```python
from build123d import *

# Parameters (mm, degrees)
F1_DEPTH = 21.6916
F3_DEPTH = 2
F0_R     = 3.175
F4_DEPTH = 2


with BuildPart() as f1:
    # F0 (on Top) → F1 (new body)
    with BuildSketch(Plane.XY):
        Polygon((-7.366008, 32.2749), (-13.577315, 21.5166), (-7.366008, 10.7583), (-13.577315, 0), (-6.788658, -11.7583), (6.788658, -11.7583), (12.999965, -1), (24.267879, -1), (30.479187, -11.7583), (44.056502, -11.7583), (50.267809, -1), (62.690424, -1), (69.479082, 10.7583), (63.267775, 21.5166), (69.479082, 32.2749), (63.267775, 43.0332), (69.479082, 53.7915), (62.690424, 65.5498), (49.113109, 65.5498), (42.901802, 54.7915), (31.633887, 54.7915), (25.42258, 65.5498), (11.845265, 65.5498), (5.633957, 54.7915), (-6.788658, 54.7915), (-13.577315, 43.0332), align=None)
        Polygon((-5.633957, 9.7583), (5.633957, 9.7583), (11.267914, 0), (5.633957, -9.7583), (-5.633957, -9.7583), (-11.267914, 0), align=None, mode=Mode.SUBTRACT)
        Polygon((11.267914, 21.5166), (5.633957, 11.7583), (-5.633957, 11.7583), (-11.267914, 21.5166), (-5.633957, 31.2749), (5.633957, 31.2749), align=None, mode=Mode.SUBTRACT)
        Polygon((12.999965, 20.5166), (24.267879, 20.5166), (29.901836, 10.7583), (24.267879, 1), (12.999965, 1), (7.366008, 10.7583), align=None, mode=Mode.SUBTRACT)
        Polygon((48.535759, 0), (42.901802, -9.7583), (31.633887, -9.7583), (25.99993, 0), (31.633887, 9.7583), (42.901802, 9.7583), align=None, mode=Mode.SUBTRACT)
        Polygon((25.99993, 21.5166), (31.633887, 31.2749), (42.901802, 31.2749), (48.535759, 21.5166), (42.901802, 11.7583), (31.633887, 11.7583), align=None, mode=Mode.SUBTRACT)
        Polygon((61.535724, 1), (50.267809, 1), (44.633852, 10.7583), (50.267809, 20.5166), (61.535724, 20.5166), (67.169681, 10.7583), align=None, mode=Mode.SUBTRACT)
        Polygon((11.267914, 43.0332), (5.633957, 33.2749), (-5.633957, 33.2749), (-11.267914, 43.0332), (-5.633957, 52.7915), (5.633957, 52.7915), align=None, mode=Mode.SUBTRACT)
        Polygon((24.267879, 22.5166), (12.999965, 22.5166), (7.366008, 32.2749), (12.999965, 42.0332), (24.267879, 42.0332), (29.901836, 32.2749), align=None, mode=Mode.SUBTRACT)
        Polygon((24.267879, 44.0332), (12.999965, 44.0332), (7.366008, 53.7915), (12.999965, 63.5498), (24.267879, 63.5498), (29.901836, 53.7915), align=None, mode=Mode.SUBTRACT)
        Polygon((25.99993, 43.0332), (31.633887, 52.7915), (42.901802, 52.7915), (48.535759, 43.0332), (42.901802, 33.2749), (31.633887, 33.2749), align=None, mode=Mode.SUBTRACT)
        Polygon((67.169681, 32.2749), (61.535724, 22.5166), (50.267809, 22.5166), (44.633852, 32.2749), (50.267809, 42.0332), (61.535724, 42.0332), align=None, mode=Mode.SUBTRACT)
        Polygon((50.267809, 63.5498), (61.535724, 63.5498), (67.169681, 53.7915), (61.535724, 44.0332), (50.267809, 44.0332), (44.633852, 53.7915), align=None, mode=Mode.SUBTRACT)
    extrude(amount=F1_DEPTH)

    # F2 (on face) → F3 (join)
    with BuildSketch(Plane(origin=(0, 0, 0), x_dir=(1, 0, 0), z_dir=(0, 0, -1))):
        Polygon((69.479082, -53.7915), (63.267775, -43.0332), (69.479082, -32.2749), (63.267775, -21.5166), (69.479082, -10.7583), (62.690424, 1), (50.267809, 1), (44.056502, 11.7583), (30.479187, 11.7583), (24.267879, 1), (12.999965, 1), (6.788658, 11.7583), (-6.788658, 11.7583), (-13.577315, 0), (-7.366008, -10.7583), (-13.577315, -21.5166), (-7.366008, -32.2749), (-13.577315, -43.0332), (-6.788658, -54.7915), (5.633957, -54.7915), (11.845265, -65.5498), (25.42258, -65.5498), (31.633887, -54.7915), (42.901802, -54.7915), (49.113109, -65.5498), (62.690424, -65.5498), align=None)
    extrude(amount=F3_DEPTH)

    # F0 (on Top) → F4 (cut, through all)
    with BuildSketch(Plane.XY):
        with Locations((0, 43.0332)):
            Circle(F0_R)
        with Locations((18.633922, 53.7915)):
            Circle(F0_R)
        with Locations((37.267844, 43.0332)):
            Circle(F0_R)
        with Locations((55.901767, 53.7915)):
            Circle(F0_R)
        with Locations((55.901767, 32.2749)):
            Circle(F0_R)
        with Locations((37.267844, 21.5166)):
            Circle(F0_R)
        with Locations((18.633922, 32.2749)):
            Circle(F0_R)
        with Locations((0, 21.5166)):
            Circle(F0_R)
        Circle(F0_R)
        with Locations((18.633922, 10.7583)):
            Circle(F0_R)
        with Locations((37.267844, 0)):
            Circle(F0_R)
        with Locations((55.901767, 10.7583)):
            Circle(F0_R)
    extrude(amount=-F4_DEPTH, mode=Mode.SUBTRACT)


solid = f1.part
```
Verification items for the finished model (mm, model axes). A direction names the side the tool comes from. Round coordinates to 2 decimals unless told otherwise and drop trailing zeros. Loops run counter-clockwise (first coordinate to the right, second up) from the corner with the lowest first, then second, coordinate; pieces in that order, holes last. Notation, with made-up numbers: (2.25, 50.25) -> (9.25, 50.25) arc R21 ccw to (9.25, 81.25) -> close; hole circle Ø7 at (-23.75, 38.5). An arc over 180 degrees is marked (long way). Answer as a JSON object with one key per item and string values.
Q1. Section check A-A (x = 0). Record the boundary of the cut face in (y, z) (1 decimal).
Data:
{"outline": "(-11.8, -2) -> (-3.2, -2) -> (-3.2, 0) -> (-9.8, 0) -> (-9.8, 21.7) -> (-11.8, 21.7) -> close; (3.2, -2) -> (18.3, -2) -> (18.3, 0) -> (11.8, 0) -> (11.8, 21.7) -> (9.8, 21.7) -> (9.8, 0) -> (3.2, 0) -> close; (24.7, -2) -> (39.9, -2) -> (39.9, 0) -> (33.3, 0) -> (33.3, 21.7) -> (31.3, 21.7) -> (31.3, 0) -> (24.7, 0) -> close; (46.2, -2) -> (54.8, -2) -> (54.8, 21.7) -> (52.8, 21.7) -> (52.8, 0) -> (46.2, 0) -> close"}
Q2. Draft check along Y on faces 5 (the flat face through (66.13, 4.96, 10.01)), 6 (the flat face through (-10.23, 48.83, 10.01)), 7 (the flat face through (37, 9.758, 11)). Enter one of: pulls with the +Y half, pulls with the -Y half, needs draft (parallel to the pull), parting line crosses it, or undercut.
Data:
{"face 5": "pulls with the -Y half", "face 6": "pulls with the +Y half", "face 7": "undercut"}
Q3. Go/stop test with flat-tipped pins: P1, Ø1, axis at y = 53, z = 5, coming from the -X side; P2, Ø5, axis at x = -0.5, z = 6, coming from the +Y side; P3, Ø12.5, axis at x = 36.5, z = 5.5, coming from the +Y side. Record where each tip stops, or that it passes through.
Data:
{"P1": "stops at x = -8.11", "P2": "stops at y = 54.79", "P3": "stops at y = 57.19"}
Q4. Access from +Z, -Z, +X, -X, +Y, -Y to the whole of each face (thin tool, end or side, straight path). Record for faces 1 (the flat face through (-8.49, 4.81, 10.69)), 2 (the flat face through (66.33, 37.73, 10.01)), 3 (the flat face through (-10.515, 26.82, 10.012)), 4 (the cylindrical face through (15.462, 10.898, -0.986)).
Data:
{"face 1": "+Z", "face 2": "+Z, -Z, +X", "face 3": "+Z, -Z, -X", "face 4": "+Z, -Z"}
Q5. Section check C-C (z = 16.5). State how many separate pieces and enclosed holes the cut face has, then the cut area to 3 significant figures.
Data:
{"separate pieces": "1", "enclosed holes": "12", "area": "1,180 mm2"}
Q6. Section check D-D (x = 18.5). Record the boundary of the cut face in (y, z).
Data:
{"outline": "(-1, -2) -> (7.59, -2) -> (7.59, 0) -> (1, 0) -> (1, 21.69) -> (-1, 21.69) -> close; (13.93, -2) -> (29.1, -2) -> (29.1, 0) -> (22.52, 0) -> (22.52, 21.69) -> (20.52, 21.69) -> (20.52, 0) -> (13.93, 0) -> close; (35.45, -2) -> (50.62, -2) -> (50.62, 0) -> (44.03, 0) -> (44.03, 21.69) -> (42.03, 21.69) -> (42.03, 0) -> (35.45, 0) -> close; (56.96, -2) -> (65.55, -2) -> (65.55, 21.69) -> (63.55, 21.69) -> (63.55, 0) -> (56.96, 0) -> close"}
Q7. Section check B-B (y = 19.5). Record the boundary of the cut face in (x, z).
Data:
{"outline": "(-12.41, -2) -> (-2.45, -2) -> (-2.45, 0) -> (-10.1, 0) -> (-10.1, 21.69) -> (-12.41, 21.69) -> close; (2.45, -2) -> (34.82, -2) -> (34.82, 0) -> (27.16, 0) -> (27.16, 21.69) -> (24.85, 21.69) -> (24.85, 0) -> (12.41, 0) -> (12.41, 21.69) -> (10.1, 21.69) -> (10.1, 0) -> (2.45, 0) -> close; (39.72, -2) -> (64.43, -2) -> (64.43, 21.69) -> (62.12, 21.69) -> (62.12, 0) -> (49.68, 0) -> (49.68, 21.69) -> (47.37, 21.69) -> (47.37, 0) -> (39.72, 0) -> close"}
Q8. Scan lines: line 1 (Y direction, x = 2, z = 12.75); line 2 (Y direction, x = 57.5, z = 1.5); line 3 (X direction, y = 43, z = 19.75). Record each from-to range of solid material in increasing order. Write a range as from..to.
Data:
{"line 1": "y = -11.76..-9.76, 9.76..11.76, 31.27..33.27, 52.79..54.79", "line 2": "y = -1..1, 20.52..22.52, 42.03..44.03, 63.55..65.55", "line 3": "x = -13.56..-11.25, 11.25..26.02, 48.52..63.29"}
